Verification items for the finished model (mm, model axes). Face numbers are marked on the shaded views. A direction names the side the tool comes from. Coordinates: 2 decimals unless noted, no trailing zeros. Write each loop counter-clockwise with the first axis right and the second up, starting at its lowest first coordinate (ties: lowest second). Pieces come first, ordered by that corner, then holes. Notation, with made-up numbers: M 31.5,45.25 L 67.5,45.25 A30 cw 67.5,83.25 Z; hole C -36,77.25 d4. An arc over 180 degrees is marked long. Answer in a Markdown table with one row per item.
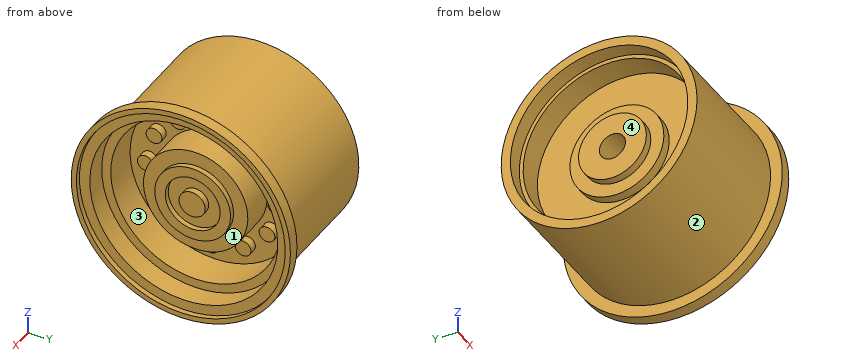
from build123d import *

# Parameters (mm, degrees)
SKETCH2_R           = 0.75
BOSS_EXTRUDE1_DEPTH = 0.75
SKETCH3_R           = 2.63
CUT_EXTRUDE1_DEPTH  = 0.5
SKETCH4_R           = 1.25
BOSS_EXTRUDE2_DEPTH = 0.6
SKETCH5_R           = 1.25
CUT_EXTRUDE2_DEPTH  = 5


with BuildPart() as part:
    # Sketch1 → Revolve2 (revolve)
    with BuildSketch(Plane.XY, mode=Mode.PRIVATE) as revolve2_sk:
        Polygon((0, 0), (-4.56, 0), (-4.56, 3.25), (-3.81, 3.25), (-3.81, 4.5), (-2.91, 4.5), (-2.91, 8.13), (-5.31, 8.13), (-5.31, 8.5), (-6.81, 8.5), (-6.81, 9.38), (5.59, 9.38), (5.59, 10.5), (6.69, 10.5), (6.69, 10), (6.19, 10), (6.19, 9), (4.19, 9), (4.19, 8.13), (0.94, 8.13), (0.94, 5), (4.19, 5), (4.19, 3.63), (4.69, 3.63), (4.69, 0), align=None)
    revolve(revolve2_sk.sketch.rotate(Axis((4.69, 0, 0), (-1, 0, 0)), 90), axis=Axis((4.69, 0, 0), (-1, 0, 0)))

    # Sketch2 → Boss-Extrude1 (add)
    with BuildSketch(Plane(origin=(0.94, 0, 0), x_dir=(0, 0, -1), z_dir=(1, 0, 0))):
        with Locations((0, 6.25)):
            Circle(SKETCH2_R)
        with Locations((3.125, 5.412658774)):
            Circle(SKETCH2_R)
        with Locations((5.412658774, 3.125)):
            Circle(SKETCH2_R)
        with Locations((6.25, 0)):
            Circle(SKETCH2_R)
        with Locations((5.412658774, -3.125)):
            Circle(SKETCH2_R)
        with Locations((3.125, -5.412658774)):
            Circle(SKETCH2_R)
        with Locations((0, -6.25)):
            Circle(SKETCH2_R)
        with Locations((-3.125, -5.412658774)):
            Circle(SKETCH2_R)
        with Locations((-5.412658774, -3.125)):
            Circle(SKETCH2_R)
        with Locations((-6.25, 0)):
            Circle(SKETCH2_R)
        with Locations((-5.412658774, 3.125)):
            Circle(SKETCH2_R)
        with Locations((-3.125, 5.412658774)):
            Circle(SKETCH2_R)
    extrude(amount=BOSS_EXTRUDE1_DEPTH)

    # Sketch3 → Cut-Extrude1 (cut)
    with BuildSketch(Plane(origin=(4.69, 0, 0), x_dir=(0, 0, -1), z_dir=(1, 0, 0))):
        Circle(SKETCH3_R)
    extrude(amount=-CUT_EXTRUDE1_DEPTH, mode=Mode.SUBTRACT)

    # Sketch4 → Boss-Extrude2 (add)
    with BuildSketch(Plane(origin=(4.19, 0, 0), x_dir=(0, 0, -1), z_dir=(1, 0, 0))):
        Circle(SKETCH4_R)
    extrude(amount=BOSS_EXTRUDE2_DEPTH)

    # Sketch5 → Cut-Extrude2 (cut)
    with BuildSketch(Plane.ZY.offset(4.56)):
        with Locations(Location((0, 0, 0), (0, 0, 180))):
            Circle(SKETCH5_R)
    extrude(amount=-CUT_EXTRUDE2_DEPTH, mode=Mode.SUBTRACT)


solid = part.part
1) Depth check by flat-ended pin: pin 1 (4 mm diameter, centred on x = 1, z = 3, fed in from -Y); pin 2 (4 mm diameter, centred on y = 0, z = 0, fed in from -X); pin 3 (1.5 mm diameter, centred on y = 7.5, z = -8, fed in from +X); pin 4 (1.5 mm diameter, centred on x = -5.5, z = 1, fed in from +Y). Enter the tip coordinate at first touch or a pass-through.
Response values:
| item | result |
|---|---|
| pin 1 | stops at y = -9.33 |
| pin 2 | stops at x = -4.56 |
| pin 3 | stops at x = 6.69 |
| pin 4 | stops at y = 9.38 |
2) Sectioned sample at B-B (x = 2.25). Record the cut outline in (y, z), then the cut area to 3 significant figures.
Response values:
| item | result |
|---|---|
| outline | C 0,0 d18.76; C 0,0 d10; hole C 0,0 d16.26 |
| area | 147 mm² |
3) Tool access check on the marked faces 3 and 4. Record the directions out of +Z, -Z, +X, -X, +Y, -Y that give a thin tool (end or side, any length) a straight path to the whole face; none if there is none.
Response values:
| item | result |
|---|---|
| face 3 | +X |
| face 4 | -X |
4) Release check for a two-part mould opening along Y. For the marked faces 1 and 2 record: +Y half, -Y half, draft (parallel to the pull), parting line (faces both ways), or undercut.
Response values:
| item | result |
|---|---|
| face 1 | undercut |
| face 2 | parting line |
5) Sectioned sample at A-A (x = -3.5). Record the cut outline in (y, z), then the cut area to 3 significant figures.
Response values:
| item | result |
|---|---|
| outline | C 0,0 d18.76; C 0,0 d9; hole C 0,0 d16.26; hole C 0,0 d2.5 |
| area | 127 mm² |
6) Thickness scan on L1, parallel to Y at x = 6.4, z = 0; L2, parallel to Y at x = 2.05, z = 0; L3, parallel to Y at x = -4.25, z = 0. Record the ranges inside material, lowest first. Write a range as [from, to].
Response values:
| item | result |
|---|---|
| L1 | y = [-10.5, -10], [10, 10.5] |
| L2 | y = [-9.38, -8.13], [-5, 5], [8.13, 9.38] |
| L3 | y = [-9.38, -8.13], [-3.25, -1.25], [1.25, 3.25], [8.13, 9.38] |
